from build123d import *

# Parameters (mm, degrees)
BOSS_EXTRUDE1_DEPTH = 7.8
SKETCH4_R           = 3.825420683
CUT_EXTRUDE2_DEPTH  = 46.305179634


with BuildPart() as part:
    # Sketch1 → Revolve1 (revolve)
    with BuildSketch(Plane.XY, mode=Mode.PRIVATE) as revolve1_sk:
        Polygon((0, 0), (0, 40.6), (4, 40.6), (6.05, 38), (6.05, 26.8), (12.7, 26.8), (12.7, 19), (9.75, 19), (9.75, 4), (7.4, 0), align=None)
    revolve(revolve1_sk.sketch.rotate(Axis((0, 0, 0), (0, 1, 0)), 90), axis=Axis((0, 0, 0), (0, 1, 0)))

    # Sketch3 → Boss-Extrude1 (add)
    with BuildSketch(Plane(origin=(0, 26.8, 0), x_dir=(1, 0, 0), z_dir=(0, 1, 0))):
        Polygon((14.224650165, -3.777575457), (10.383801393, 10.430120675), (-3.840848772, 14.207696132), (-14.224650165, 3.777575457), (-10.383801393, -10.430120675), (3.840848772, -14.207696132), align=None)
    extrude(amount=-BOSS_EXTRUDE1_DEPTH)

    # Sketch4 → Cut-Extrude2 (cut, through all)
    with BuildSketch(Plane(origin=(0, 40.6, 0), x_dir=(1, 0, 0), z_dir=(0, 1, 0))):
        with Locations(Location((0, 0, 0), (0, 0, 270))):
            Circle(SKETCH4_R)
    extrude(amount=-CUT_EXTRUDE2_DEPTH, mode=Mode.SUBTRACT)


solid = part.part
Design review of the part built by this model. Coordinates are the model's own, in mm. A direction names the side the tool comes from. Give positions to 0.01 mm unless a question says otherwise; leave off trailing zeros. Write each loop counter-clockwise with the first axis right and the second up, starting at its lowest first coordinate (ties: lowest second). Pieces come first, ordered by that corner, then holes. Notation, with made-up numbers: M -31.75,51.25 L -21.75,51.25 A24 ccw -21.75,62.25 Z; hole C -37.5,69 d7. An arc over 180 degrees is marked long. Answer as a JSON object with one key per item and string values. Group by question number.
1) Clearance check with flat-ended pins moving along their axes: pin 1 Ø10 at (x, y) = (0, 12) entering from -Z; pin 2 Ø4 at (x, y) = (7.5, 35) entering from +Z; pin 3 Ø1 at (y, z) = (11, -5) entering from +X. State where each tip first meets the part, or that it passes through.
2) We need section B-B (x = 0). Give the boundary of the cut face in (y, z).
3) Mouldability with a two-part tool opening along Z and no side actions: class faces 1 (the face through (-9.667, 11.395, 1.269)), 2 (the face through (-3.734, 20.584, -0.829)), 3 (the face through (-8.96, 22.955, -9.066)) as released by +Z, released by -Z, zero draft, split by the parting line, or undercut.
4) For line 1 along X through (y, z) = (30, 0); line 2 along X through (y, z) = (10.5, 0); line 3 along Y through (x, z) = (-0.5, -10), list the stretches that pass through material, from the lowest coordinate up.
5) Tool access review of faces 4 (the face through (2, 19, -10)), 5 (the face through (-1.82, 32.32, -5.77)), 6 (the face through (-12.33, 22.95, 3.23)): name each direction out of +Z, -Z, +X, -X, +Y, -Y from which nothing blocks a thin tool from reaching the whole face with its end or side.
6) We need section C-C (z = 0). Give the boundary of the cut face in (x, y), and give its area (3 significant figures).
7) We need section A-A (y = 22.5). Give the boundary of the cut face in (x, z), and give its area (3 significant figures).
8) We need section D-D (y = 7). Give the boundary of the cut face in (x, z), and give its area (3 significant figures).
Answer key:
{
 "1": {"pin 1": "stops at z = -9.75", "pin 2": "stops at z = 2.52", "pin 3": "stops at x = 8.65"},
 "2": {"outline": "M 0,-7.4 L 4,-9.75 L 19,-9.75 L 19,-13.19 L 26.8,-13.19 L 26.8,-6.05 L 38,-6.05 L 40.6,-4 L 40.6,-3.83 L 0,-3.83 Z; M 0,3.83 L 40.6,3.83 L 40.6,4 L 38,6.05 L 26.8,6.05 L 26.8,13.19 L 19,13.19 L 19,9.75 L 4,9.75 L 0,7.4 Z"},
 "3": {"face 1": "split by the parting line", "face 2": "undercut", "face 3": "released by -Z"},
 "4": {"line 1": "x = -6.05 to -3.83, 3.83 to 6.05", "line 2": "x = -9.75 to -3.83, 3.83 to 9.75", "line 3": "y = 19 to 26.8"},
 "5": {"face 4": "-Y", "face 5": "+Y", "face 6": "+Z, -X, +Y, -Y"},
 "6": {"outline": "M -13.2,19 L -9.75,19 L -9.75,4 L -7.4,0 L -3.83,0 L -3.83,40.6 L -4,40.6 L -6.05,38 L -6.05,26.8 L -13.2,26.8 Z; M 3.83,0 L 7.4,0 L 9.75,4 L 9.75,19 L 13.2,19 L 13.2,26.8 L 6.05,26.8 L 6.05,38 L 4,40.6 L 3.83,40.6 Z", "area": "418 mm²"},
 "7": {"outline": "M -14.22,-3.78 L -3.84,-14.21 L 10.38,-10.43 L 14.22,3.78 L 3.84,14.21 L -10.38,10.43 Z; hole C 0,0 d7.65", "area": "517 mm²"},
 "8": {"outline": "C 0,0 d19.5; hole C 0,0 d7.65", "area": "253 mm²"}
}
